from build123d import *

# Parameters (mm, degrees)
ESQUISSE1_W                                = 70
ESQUISSE1_H                                = 46
BOSS_EXTRU_1_DEPTH                         = 5
D_GAGEMENT_M51_D                           = 5.5
D_GAGEMENT_M41_D                           = 4.5
CHAMBRAGE_POUR_VIS_T_TE_RONDE_BOMB_2_COUNT = 2
CHAMBRAGE_POUR_VIS_T_TE_RONDE_BOMB_2_PITCH = 20
CHAMBRAGE_POUR_VIS_T_TE_RONDE_BOMB_3_COUNT = 2
CHAMBRAGE_POUR_VIS_T_TE_RONDE_BOMB_3_PITCH = 28.284271247
CHAMBRAGE_POUR_VIS_T_TE_RONDE_BOMB_4_COUNT = 2
CHAMBRAGE_POUR_VIS_T_TE_RONDE_BOMB_4_PITCH = 20


with BuildPart() as part:
    # Esquisse1 → Boss.-Extru.1 (new body)
    with BuildSketch(Plane.XY):
        Rectangle(ESQUISSE1_W, ESQUISSE1_H)
    extrude(amount=BOSS_EXTRU_1_DEPTH)

    # Dégagement M51 (through all)
    with Locations(Plane.XY.offset(5)):
        with Locations((22.5, -17.116426572), (22.5, 16.883573428), (-22.5, 16.883573428), (-22.5, -17.116426572)):
            Hole(D_GAGEMENT_M51_D / 2)

    # Dégagement M41 (through all)
    with Locations(Plane(origin=(0, 0, 0), x_dir=(-1, 0, 0), z_dir=(0, 0, -1))):
        with Locations((10, -10), (-10, -10), (-10, 10), (10, 10)):
            Hole(D_GAGEMENT_M41_D / 2)

    # Esquisse6 → Chambrage pour vis à tête ronde bombée M41 (revolve, cut)
    with BuildSketch(Plane(origin=(-10, -10, 5), x_dir=(0, -1, 0), z_dir=(1, 0, 0))):
        Polygon((0, 0), (0, 5), (2.25, 5), (2.25, 3.125), (2.275, 3.1), (4.5, 3.1), (4.5, 0), align=None)
    chambrage_pour_vis_t_te_ronde_bomb_e_m = revolve(axis=Axis((-10, -10, 11.35), (0, 0, -1)), mode=Mode.SUBTRACT)

    # Chambrage pour vis _ t_te ronde bomb 2: Chambrage pour vis à tête ronde bombée M41 ×2
    with Locations(*[(0, i * CHAMBRAGE_POUR_VIS_T_TE_RONDE_BOMB_2_PITCH, 0) for i in range(1, CHAMBRAGE_POUR_VIS_T_TE_RONDE_BOMB_2_COUNT)]):
        add(chambrage_pour_vis_t_te_ronde_bomb_e_m, mode=Mode.SUBTRACT)

    # Chambrage pour vis _ t_te ronde bomb 3: Chambrage pour vis à tête ronde bombée M41 ×2
    with Locations(*[Vector(0.7071067811865407, 0.7071067811865545, 0) * (i * CHAMBRAGE_POUR_VIS_T_TE_RONDE_BOMB_3_PITCH) for i in range(1, CHAMBRAGE_POUR_VIS_T_TE_RONDE_BOMB_3_COUNT)]):
        add(chambrage_pour_vis_t_te_ronde_bomb_e_m, mode=Mode.SUBTRACT)

    # Chambrage pour vis _ t_te ronde bomb 4: Chambrage pour vis à tête ronde bombée M41 ×2
    with Locations(*[(i * CHAMBRAGE_POUR_VIS_T_TE_RONDE_BOMB_4_PITCH, 0, 0) for i in range(1, CHAMBRAGE_POUR_VIS_T_TE_RONDE_BOMB_4_COUNT)]):
        add(chambrage_pour_vis_t_te_ronde_bomb_e_m, mode=Mode.SUBTRACT)


solid = part.part
The listing builds one solid part. Answer for the finished solid, in the listing's coordinates (mm). A direction names the side the tool comes from. Round coordinates to 2 decimals unless told otherwise and drop trailing zeros. Write each loop counter-clockwise with the first axis right and the second up, starting at its lowest first coordinate (ties: lowest second). Pieces come first, ordered by that corner, then holes. Notation, with made-up numbers: (19.5, 60.5) - (54.5, 60.5) arc R15 cw to (54.5, 68.5) - close; hole circle Ø1 at (2.25, 42). An arc over 180 degrees is marked (long way). Use a Markdown table: item, result. Add a question column.
1. The part is cut by section D-D (x = 23.5). Write down the section's boundary in (y, z).
2. For a pull along X with two mould halves and no side action, classify faces 3 (the face through (-35, 0, 2)), 4 (the face through (-11.66, 11.52, 0.95)), 5 (the face through (0, 0, 0)) as +X half, -X half, draft (parallel to the pull), parting line (faces both ways), or undercut.
3. Consider line 1 (Y direction, x = 10, z = 3.5); line 2 (X direction, y = 10, z = 3.75); line 3 (X direction, y = -10, z = 0.95). Determine where each line is inside the solid, lowest interval first.
4. The part is cut by section B-B (y = 10). Write down the section's boundary in (x, z) (3 decimals), and give its area (3 significant figures).
5. The part is cut by section C-C (z = 3.05). Give the number of separate pieces and of enclosed holes in the cut face, and give its area (3 significant figures).
6. The part is cut by section A-A (x = 10). Write down the section's boundary in (y, z) (3 decimals), and give its area (3 significant figures).
7. Flat-ended cylindrical pins translate along their axes: P1, Ø4, axis at x = -21, y = -9.5, coming from the -Z side; P2, Ø4, axis at x = -10, y = -10, coming from the +Z side; P3, Ø6, axis at x = 10, y = 10, coming from the +Z side. Find the tip coordinate at first contact, or state that the pin passes through.
8. A tool of negligible diameter and unlimited length cuts with its end or side. For faces 1 (the face through (12, 12, 1.9)), 2 (the face through (-11.66, -8.48, 0.95)), from which of +Z, -Z, +X, -X, +Y, -Y can it reach the whole face along a straight path? Write none if from no direction.
Reported:
| question | item | result |
|---|---|---|
| 1 | outline | (-23, 0) - (-19.68, 0) - (-19.68, 5) - (-23, 5) - close; (-14.55, 0) - (14.32, 0) - (14.32, 5) - (-14.55, 5) - close; (19.45, 0) - (23, 0) - (23, 5) - (19.45, 5) - close |
| 2 | face 3 | -X half |
| 2 | face 4 | undercut |
| 2 | face 5 | draft |
| 3 | line 1 | -23 to -14.5, -5.5 to 5.5, 14.5 to 23 |
| 3 | line 2 | -35 to -14.5, -5.5 to 5.5, 14.5 to 35 |
| 3 | line 3 | -35 to -12.25, -7.75 to 7.75, 12.25 to 35 |
| 4 | outline | (-35, 0) - (-12.25, 0) - (-12.25, 1.875) - (-12.275, 1.9) - (-14.5, 1.9) - (-14.5, 5) - (-35, 5) - close; (-7.75, 0) - (7.75, 0) - (7.75, 1.875) - (7.725, 1.9) - (5.5, 1.9) - (5.5, 5) - (-5.5, 5) - (-5.5, 1.9) - (-7.725, 1.9) - (-7.75, 1.875) - close; (12.25, 0) - (35, 0) - (35, 5) - (14.5, 5) - (14.5, 1.9) - (12.275, 1.9) - (12.25, 1.875) - close |
| 4 | area | 277 mm^2 |
| 5 | separate pieces | 1 |
| 5 | enclosed holes | 8 |
| 5 | area | 2,870 mm^2 |
| 6 | outline | (-23, 0) - (-12.25, 0) - (-12.25, 1.875) - (-12.275, 1.9) - (-14.5, 1.9) - (-14.5, 5) - (-23, 5) - close; (-7.75, 0) - (7.75, 0) - (7.75, 1.875) - (7.725, 1.9) - (5.5, 1.9) - (5.5, 5) - (-5.5, 5) - (-5.5, 1.9) - (-7.725, 1.9) - (-7.75, 1.875) - close; (12.25, 0) - (23, 0) - (23, 5) - (14.5, 5) - (14.5, 1.9) - (12.275, 1.9) - (12.25, 1.875) - close |
| 6 | area | 157 mm^2 |
| 7 | P1 | z = 0 |
| 7 | P2 | through |
| 7 | P3 | z = 1.9 |
| 8 | face 1 | +Z |
| 8 | face 2 | +Z, -Z |
